Work out the finished part from the listing and answer in its coordinate system (mm). Face numbers are marked on the shaded views. A direction names the side the tool comes from. Give positions to 0.01 mm unless a question says otherwise; leave off trailing zeros. Order: outer loops, then holes, each group sorted by start corner. A loop starts at its lowest first (then second) coordinate and runs counter-clockwise, first axis right, second up. Notation, with made-up numbers: (-9.75, -24.5) - (49.25, -24.5) arc R22 ccw to (49.25, 12.5) - close; hole circle Ø8 at (21.5, -20). An arc over 180 degrees is marked (long way). Return JSON: item names as keys, results as strings. Group by question number.
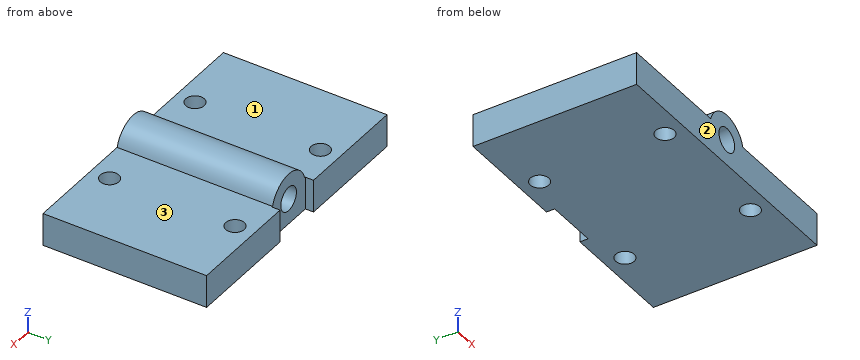
from build123d import *

# Parameters (mm, degrees)
EXTRUDE_1_DEPTH             = 28.5
SKETCH_2_W                  = 20.65
SKETCH_2_H                  = 6
EXTRUDE_2_DEPTH             = 1.5
SKETCH_3_W                  = 20.65
SKETCH_3_H                  = 6
EXTRUDE_3_DEPTH             = 1.5
HOLE_WIZARD_4_4_4_4_1_D     = 4.4
HOLE_WIZARD_4_4_4_4_1_DEPTH = 28.5
HOLE_WIZARD_3_4_3_4_1_D     = 3.4
HOLE_WIZARD_3_4_3_4_1_DEPTH = 9.4


with BuildPart() as part:
    # 草图1 → 凸台-拉伸1 (new body)
    with BuildSketch(Plane(origin=(0, 253.5, 0), x_dir=(1, 0, 0), z_dir=(0, 1, 0))):
        with BuildLine():
            Line((264.516635916, -508.1), (285.35, -508.1))
            Line((285.35, -508.1), (285.35, -502.1))
            Line((285.35, -502.1), (234.65, -502.1))
            Line((234.65, -502.1), (234.65, -508.1))
            Line((234.65, -508.1), (255.483364084, -508.1))
            ThreePointArc((255.483364084, -508.1), (260, -511.5), (264.516635916, -508.1))
        make_face()
    extrude(amount=-EXTRUDE_1_DEPTH)

    # 草图2 → 凸台-拉伸2 (add)
    with BuildSketch(Plane(origin=(0, 253.5, 0), x_dir=(-1, 0, 0), z_dir=(0, 1, 0))):
        with Locations((-275.025, 505.1)):
            Rectangle(SKETCH_2_W, SKETCH_2_H)
    extrude(amount=EXTRUDE_2_DEPTH)

    # 草图3 → 凸台-拉伸3 (add)
    with BuildSketch(Plane(origin=(0, 253.5, 0), x_dir=(-1, 0, 0), z_dir=(0, 1, 0))):
        with Locations((-244.975, 505.1)):
            Rectangle(SKETCH_3_W, SKETCH_3_H)
    extrude(amount=EXTRUDE_3_DEPTH)

    # Ø4.4 (4.4) 直径孔1
    with Locations(Plane(origin=(0, 253.5, 0), x_dir=(1, 0, 0), z_dir=(0, 1, 0))):
        with Locations((260, -506.8)):
            Hole(HOLE_WIZARD_4_4_4_4_1_D / 2, depth=HOLE_WIZARD_4_4_4_4_1_DEPTH)

    # Ø3.4 (3.4) 直径孔1
    with Locations(Plane(origin=(0, 0, 502.1), x_dir=(-1, 0, 0), z_dir=(0, 0, -1))):
        with Locations((-248, 228.5), (-248, 251.5), (-272, 251.5), (-272, 228.5)):
            Hole(HOLE_WIZARD_3_4_3_4_1_D / 2, depth=HOLE_WIZARD_3_4_3_4_1_DEPTH)


solid = part.part
1. Consider probe 1 along X at (y, z) = (251.5, 506.85); probe 2 along Y at (x, z) = (272, 506.9); probe 3 along X at (y, z) = (229.5, 506.25). Determine where each line is inside the solid, lowest interval first. Write a range as from..to.
2. The part is cut by section B-B (y = 228.5). Give the vertices of the cut face in (x, z).
3. The part is cut by section C-C (x = 272). Give the vertices of the cut face in (y, z), and give its area (3 significant figures).
4. The part is cut by section A-A (z = 506.8). Give the vertices of the cut face in (x, y), and give its area (3 significant figures).
5. Each of these flat-tipped pins is pushed along its axis until it touches: pin 1 (4.5 mm diameter, centred on x = 248, y = 251.5, fed in from -Z); pin 2 (1.5 mm diameter, centred on x = 268.5, z = 509, fed in from +Y); pin 3 (1 mm diameter, centred on x = 278.5, y = 236, fed in from +Z). Where does it stop, or does it pass through?
6. A tool of negligible diameter and unlimited length cuts with its end or side. For the marked faces 1, 2 and 3, from which of +Z, -Z, +X, -X, +Y, -Y can it reach the whole face along a straight path? Write none if from no direction.
7. The part is cut by section D-D (y = 246.25). Give the vertices of the cut face in (x, z), and give its area (3 significant figures).
Answers:
{
 "1": {"probe 1": "x = 234.65..246.3, 249.7..257.8, 262.2..270.3, 273.7..285.35", "probe 2": "y = 225..226.8, 230.2..249.8, 253.2..255", "probe 3": "x = 234.65..246.63, 249.37..257.87, 262.13..270.63, 273.37..285.35"},
 "2": {"outline": "(234.65, 502.1) - (246.3, 502.1) - (246.3, 508.1) - (234.65, 508.1) - close; (249.7, 502.1) - (270.3, 502.1) - (270.3, 508.1) - (264.52, 508.1) arc R4.7 ccw to (255.48, 508.1) - (249.7, 508.1) - close; (273.7, 502.1) - (285.35, 502.1) - (285.35, 508.1) - (273.7, 508.1) - close; hole circle Ø4.4 at (260, 506.8)"},
 "3": {"outline": "(225, 502.1) - (226.8, 502.1) - (226.8, 508.1) - (225, 508.1) - close; (230.2, 502.1) - (249.8, 502.1) - (249.8, 508.1) - (230.2, 508.1) - close; (253.2, 502.1) - (255, 502.1) - (255, 508.1) - (253.2, 508.1) - close", "area": "139 mm^2"},
 "4": {"outline": "(234.65, 225) - (257.8, 225) - (257.8, 253.5) - (255.3, 253.5) - (255.3, 255) - (234.65, 255) - close; (262.2, 225) - (285.35, 225) - (285.35, 255) - (264.7, 255) - (264.7, 253.5) - (262.2, 253.5) - close; hole circle Ø3.4 at (248, 228.5); hole circle Ø3.4 at (248, 251.5); hole circle Ø3.4 at (272, 228.5); hole circle Ø3.4 at (272, 251.5)", "area": "1,350 mm^2"},
 "5": {"pin 1": "stops at z = 502.1", "pin 2": "passes through", "pin 3": "stops at z = 508.1"},
 "6": {"face 1": "+Z, -X, +Y, -Y", "face 2": "+Z, -Z, +X, -X, -Y", "face 3": "+Z, +X, +Y, -Y"},
 "7": {"outline": "(234.65, 502.1) - (285.35, 502.1) - (285.35, 508.1) - (264.52, 508.1) arc R4.7 ccw to (255.48, 508.1) - (234.65, 508.1) - close; hole circle Ø4.4 at (260, 506.8)", "area": "312 mm^2"}
}
